from build123d import *

# Parameters (mm, degrees)
SKETCH1_W           = 134
SKETCH1_H           = 50
BOSS_EXTRUDE1_DEPTH = 3
SKETCH2_W           = 94
SKETCH2_H           = 40
CUT_EXTRUDE1_DEPTH  = 13
SKETCH3_W           = 10
SKETCH3_H           = 3
BOSS_EXTRUDE2_DEPTH = 3


with BuildPart() as part:
    # Sketch1 → Boss-Extrude1 (new body)
    with BuildSketch(Plane(origin=(0, 0, 0), x_dir=(1, 0, 0), z_dir=(0, 1, 0))):
        Rectangle(SKETCH1_W, SKETCH1_H)
    extrude(amount=BOSS_EXTRUDE1_DEPTH)

    # Sketch2 → Cut-Extrude1 (cut)
    with BuildSketch(Plane(origin=(0, 3, 0), x_dir=(1, 0, 0), z_dir=(0, 1, 0))):
        with Locations((0, -5)):
            Rectangle(SKETCH2_W, SKETCH2_H)
    extrude(amount=-CUT_EXTRUDE1_DEPTH, mode=Mode.SUBTRACT)

    # Sketch3 → Boss-Extrude2 (add)
    with BuildSketch(Plane(origin=(0, 0, -25), x_dir=(-1, 0, 0), z_dir=(0, 0, -1))):
        with Locations((-45, 1.5)):
            Rectangle(SKETCH3_W, SKETCH3_H)
        with Locations((-15, 1.5)):
            Rectangle(SKETCH3_W, SKETCH3_H)
        with Locations((15, 1.5)):
            Rectangle(SKETCH3_W, SKETCH3_H)
        with Locations((45, 1.5)):
            Rectangle(SKETCH3_W, SKETCH3_H)
    extrude(amount=BOSS_EXTRUDE2_DEPTH)


solid = part.part
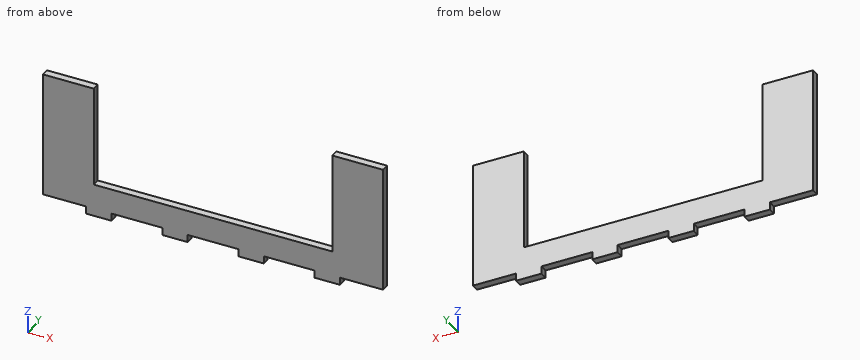
Model file for the job. Use its own axes, mm. Coordinates: 2 decimals unless noted, no trailing zeros. Order: outer loops, then holes, each group sorted by start corner. A loop starts at its lowest first (then second) coordinate and runs counter-clockwise, first axis right, second up. Notation, with made-up numbers: (-37, 29) -> (-32, 29) arc R17 cw to (-32, 54) -> close; hole circle Ø4 at (-35, -33). An arc over 180 degrees is marked (long way). Return JSON: item names as keys, results as strings. Group by question number.
Item 1: Flat gauge pins, fed straight in: P1, Ø0.9, axis at y = 2, z = -26.5, coming from the -X side; P2, Ø0.9, axis at y = 2, z = -26.5, coming from the +X side; P3, Ø0.9, axis at x = -25.5, y = 2, coming from the -Z side. Where does each tip first touch, or does it go through?
Item 2: Saw through at B-B on y = 0.75. Write the cut outline in (x, z).
Item 3: Wall check: line 1 along X through (y, z) = (1.5, -12); line 2 along Z through (x, y) = (21, 1.2); line 3 along Z through (x, y) = (54, 0.8). Give the ranges that are in metal, low to high. Write a range as [from, to].
Item 4: Saw through at C-C on x = -17. Write the cut outline in (y, z).
Item 5: Saw through at A-A on z = -2.5. Write the cut outline in (x, y).
Item 6: Saw through at D-D on x = -51.5. Write the cut outline in (y, z), then the cut area to 3 significant figures.
Values found:
{
 "1": {"P1": "stops at x = -50", "P2": "stops at x = 50", "P3": "stops at z = -25"},
 "2": {"outline": "(-67, -25) -> (-50, -25) -> (-50, -28) -> (-40, -28) -> (-40, -25) -> (-20, -25) -> (-20, -28) -> (-10, -28) -> (-10, -25) -> (10, -25) -> (10, -28) -> (20, -28) -> (20, -25) -> (40, -25) -> (40, -28) -> (50, -28) -> (50, -25) -> (67, -25) -> (67, 25) -> (47, 25) -> (47, -15) -> (-47, -15) -> (-47, 25) -> (-67, 25) -> close"},
 "3": {"line 1": "x = [-67, -47], [47, 67]", "line 2": "z = [-25, -15]", "line 3": "z = [-25, 25]"},
 "4": {"outline": "(0, -28) -> (3, -28) -> (3, -15) -> (0, -15) -> close"},
 "5": {"outline": "(-67, 0) -> (-47, 0) -> (-47, 3) -> (-67, 3) -> close; (47, 0) -> (67, 0) -> (67, 3) -> (47, 3) -> close"},
 "6": {"outline": "(0, -25) -> (3, -25) -> (3, 25) -> (0, 25) -> close", "area": "150 mm2"}
}
